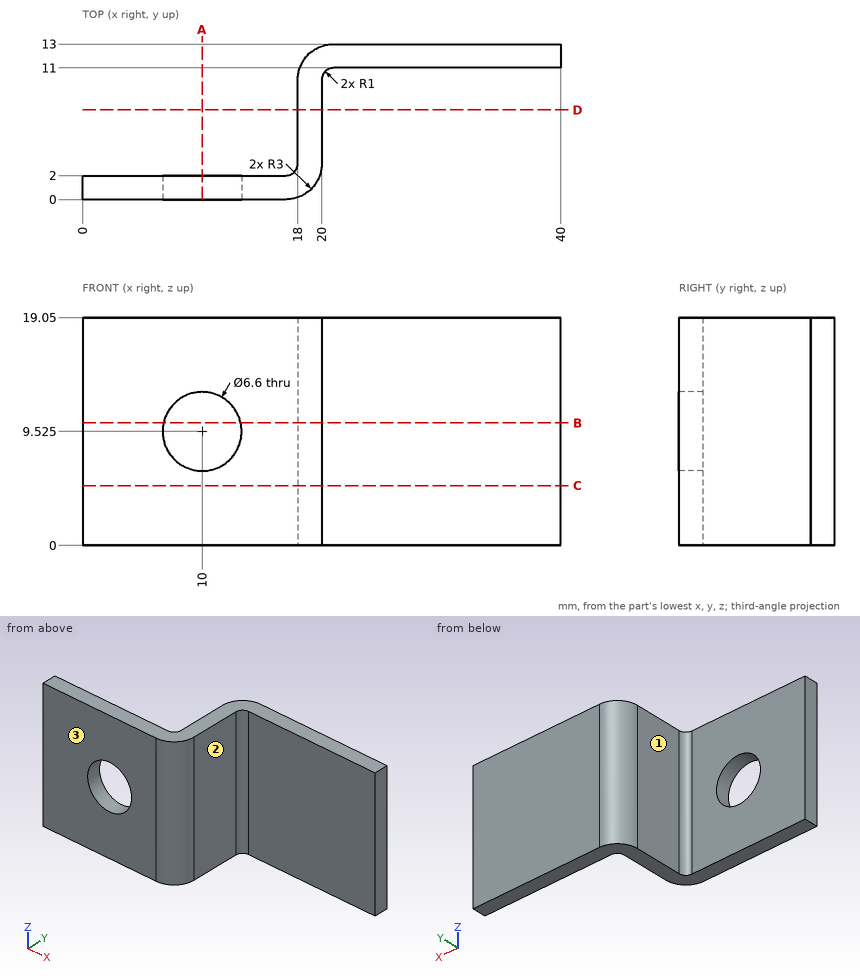
The figure shows three views and two pictorial views of one solid part (mm, origin at its lowest corner). Answer the questions. A direction names the side the tool comes from. Give positions to 0.01 mm unless a question says otherwise; leave off trailing zeros. Loops run counter-clockwise (first coordinate to the right, second up) from the corner with the lowest first, then second, coordinate; pieces in that order, holes last. Notation, with made-up numbers: (-29.5, -18) -> (11.5, -18) arc R27 ccw to (11.5, 18) -> close; hole circle Ø3 at (85, 86). An arc over 180 degrees is marked (long way). Put each result on its own line as item: value. Start each with the question number.
Item 1: The part is cut by section D-D (y = 7.5). Give the vertices of the cut face in (x, z), then the cut area to 3 significant figures.
Item 2: The part is cut by section A-A (x = 10). Give the vertices of the cut face in (y, z) (3 decimals), then the cut area to 3 significant figures.
Item 3: Which of the six approach directions +Z, -Z, +X, -X, +Y, -Y give full straight-line access (tool end or side, diameter ignored) to the marked faces 1, 2 and 3?
Item 4: Find the intervals of material crossed by L1, parallel to Z at x = 10, y = 1.25 (3 decimals); L2, parallel to X at y = 8.5, z = 8.75; L3, parallel to Y at x = 24.5, z = 17.25, in increasing order. Write a range as [from, to].
Item 5: The part is cut by section B-B (z = 10.25). Give the vertices of the cut face in (x, y).
Item 6: Each of these flat-tipped pins is pushed along its axis until it touches: P1, Ø2, axis at y = 8, z = 14, coming from the -X side; P2, Ø8.5, axis at x = 7.5, z = 14, coming from the +Y side; P3, Ø1.5, axis at y = 9.5, z = 10.5, coming from the +X side. Where does it stop, or does it pass through?
Item 7: The part is cut by section C-C (z = 5). Give the vertices of the cut face in (x, y).
Answers below:
1. outline: (18, 0) -> (20, 0) -> (20, 19.05) -> (18, 19.05) -> close
1. area: 38.1 mm2
2. outline: (0, 0) -> (2, 0) -> (2, 6.225) -> (0, 6.225) -> close; (0, 12.825) -> (2, 12.825) -> (2, 19.05) -> (0, 19.05) -> close
2. area: 24.9 mm2
3. face 1: +Z, -Z, -X, +Y
3. face 2: +Z, -Z, +X, -Y
3. face 3: +Z, -Z, +X, -X, -Y
4. L1: [0, 6.225], [12.825, 19.05]
4. L2: [18, 20]
4. L3: [11, 13]
5. outline: (0, 0) -> (6.78, 0) -> (6.78, 2) -> (0, 2) -> close; (13.22, 0) -> (17, 0) arc R3 ccw to (20, 3) -> (20, 10) arc R1 cw to (21, 11) -> (40, 11) -> (40, 13) -> (21, 13) arc R3 ccw to (18, 10) -> (18, 3) arc R1 cw to (17, 2) -> (13.22, 2) -> close
6. P1: x = 18
6. P2: y = 2
6. P3: x = 20.03
7. outline: (0, 0) -> (17, 0) arc R3 ccw to (20, 3) -> (20, 10) arc R1 cw to (21, 11) -> (40, 11) -> (40, 13) -> (21, 13) arc R3 ccw to (18, 10) -> (18, 3) arc R1 cw to (17, 2) -> (0, 2) -> close
